The model under review builds one solid part; all positions refer to its coordinate system, in mm. Face numbers are marked on the shaded views. A direction names the side the tool comes from. Round coordinates to 2 decimals unless told otherwise and drop trailing zeros. Loops run counter-clockwise (first coordinate to the right, second up) from the corner with the lowest first, then second, coordinate; pieces in that order, holes last. Notation, with made-up numbers: (-28, 69.25) -> (2, 69.25) arc R20 cw to (2, 73.25) -> close; hole circle Ø11 at (84.5, 5.5). An arc over 180 degrees is marked (long way). Return JSON: item names as keys, results as strings. Group by question number.
Autodesk Inventor part; units mm, degrees
ref_plane "YZ Plane" through (0, 0, 0) normal (1, 0, 0) x (0, 1, 0)
ref_plane "XZ Plane" through (0, 0, 0) normal (0, 1, 0) x (-1, 0, 0)
ref_plane "XY Plane" through (0, 0, 0) normal (0, 0, 1) x (1, 0, 0)
sketch "Эскиз1" plane through (0, 0, 0) normal (0, 0, 1) x (1, 0, 0)
  circle A0 centre (0, 0) radius 3.25
  circle A1 centre (0, 0) radius 4.5
  dimension "d0" = 6.5
  dimension "d1" = 9
extrude "Выдавливание1" add sketch "Эскиз1" along normal blind 5.25
sketch "Эскиз2" plane through (0, 0, 0) normal (0, 0, -1) x (-1, 0, 0)
  circle A0 centre (0, 0) radius 5.5
  dimension "d4" = 11
loft "Лофт1" add profiles "Эскиз2" section 2 edges at (-4.5, 0, 5.25)
sketch "Эскиз4" plane through (0, 0, 0) normal (0, 0, -1) x (-1, 0, 0)
  circle A0 centre (0, 0) radius 3.25
  dimension "d10" = 6.5
extrude "Выдавливание2" cut sketch "Эскиз4" against normal through all
sketch "Эскиз5" plane through (0, 0, 0) normal (0, 0, -1) x (-1, 0, 0)
  circle A0 centre (-8.8669, 1.5421) radius 2.1
  circle A1 centre (-1.5421, -8.8669) radius 2.1
  circle A2 centre (1.5421, 8.8669) radius 2.1
  circle A3 centre (8.8669, -1.5421) radius 2.1
  circle A4 centre (0, 0) radius 13.5
  circle A5 centre (0, 0) radius 3.25
  dimension "d13" = 27
extrude "Выдавливание3" add sketch "Эскиз5" against normal blind 3
fillet "Сопряжение1" radius 2 1 edges at (4.9286, 0, 3)
chamfer "Фаска1" distance 2 angle 45 4 edges at (0.5579, 8.8669, 3) (10.9669, 1.5421, 3) (-6.7669, -1.5421, 3) (3.6421, -8.8669, 3)
sketch "Эскиз6" plane through (0, 0, 0) normal (0, 0, -1) x (-1, 0, 0)
  circle A0 centre (0, 0) radius 13.5
  circle A1 centre (8.8669, -1.5421) radius 2.1
  circle A2 centre (1.5421, 8.8669) radius 2.1
  circle A3 centre (-1.5421, -8.8669) radius 2.1
  circle A4 centre (-8.8669, 1.5421) radius 2.1
  circle A5 centre (0, 0) radius 3.25
extrude "Выдавливание4" add sketch "Эскиз6" against normal blind 3
sketch "Эскиз8" plane through (0, 0, 3) normal (0, 0, 1) x (1, 0, 0)
  point P0 (0, 0)
sketch "Эскиз9" plane through (0, 0, 5.25) normal (0, 0, 1) x (1, 0, 0)
  circle A0 centre (0, 0) radius 4.5
  circle A1 centre (0, 0) radius 3.25
extrude "Выдавливание6" add sketch "Эскиз9" along normal blind 3.75
properties part number "втулка для крепл 3" material "Пластик ПЭТ"
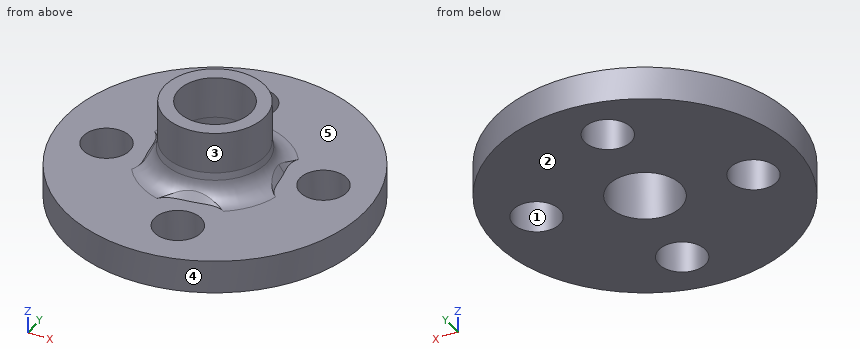
1. For P1, Ø3, axis at y = -7, z = 1, coming from the -X side; P2, Ø2, axis at x = 9, z = 1.5, coming from the -Y side; P3, Ø4, axis at x = -8, z = 2, coming from the -Y side, all flat-tipped, find the tip position at first contact; note any pin that passes through.
2. We need section C-C, the plane z = 1.5. Write out the cut boundary in (x, y), then the cut area to 3 significant figures.
3. We need section A-A, the plane z = 6.5. Write out the cut boundary in (x, y).
4. Tool access review of the marked faces 4 and 5: name each direction out of +Z, -Z, +X, -X, +Y, -Y from which nothing blocks a thin tool from reaching the whole face with its end or side.
5. We need section B-B, the plane x = -8.5. Write out the cut boundary in (y, z), then the cut area to 3 significant figures.
6. Draft analysis for pull direction X (two halves, no side actions). For the marked faces 1, 2 and 3, state which applies: pulls with the +X half, pulls with the -X half, needs draft (parallel to the pull), parting line crosses it, or undercut.
7. We need section D-D, the plane x = 0. Give the number of separate pieces and of enclosed holes in the cut face, then the cut area to 3 significant figures.
8. Wall thickness on line 1 (Z direction, x = 2.25, y = 4.5); line 2 (X direction, y = 0.25, z = 3.5); line 3 (Z direction, x = 7.5, y = -4): over which ranges is each line inside the solid? List them lowest first.
Check sheet entries:
{
 "1": {"P1": "stops at x = -12.33", "P2": "stops at y = -10.87", "P3": "stops at y = -12.09"},
 "2": {"outline": "circle Ø27 at (0, 0); hole circle Ø4.2 at (-8.87, -1.54); hole circle Ø4.2 at (-1.54, 8.87); hole circle Ø6.5 at (0, 0); hole circle Ø4.2 at (1.54, -8.87); hole circle Ø4.2 at (8.87, 1.54)", "area": "484 mm²"},
 "3": {"outline": "circle Ø9 at (0, 0); hole circle Ø6.5 at (0, 0)"},
 "4": {"face 4": "+Z, -Z", "face 5": "+Z"},
 "5": {"outline": "(-10.49, 0) -> (-3.61, 0) -> (-3.61, 3) -> (-10.49, 3) -> close; (0.53, 0) -> (10.49, 0) -> (10.49, 3) -> (0.53, 3) -> close", "area": "50.5 mm²"},
 "6": {"face 1": "undercut", "face 2": "needs draft", "face 3": "parting line crosses it"},
 "7": {"separate pieces": "4", "enclosed holes": "0", "area": "61.2 mm²"},
 "8": {"line 1": "z = 0 to 3.74", "line 2": "x = -5.25 to -3.24, 3.24 to 5.2", "line 3": "z = 0 to 3"}
}
